Check sheet for the modelled part. Datum: model origin and axes. Units: mm. Face numbers are marked on the shaded views. A direction names the side the tool comes from. Coordinates: 2 decimals unless noted, no trailing zeros. Order: outer loops, then holes, each group sorted by start corner. A loop starts at its lowest first (then second) coordinate and runs counter-clockwise, first axis right, second up.
1. Thickness scan on line 1 (X direction, y = 1.75, z = 6.25); line 2 (X direction, y = -1.5, z = 2.75) (3 decimals); line 3 (Y direction, x = -7.25, z = 4). Record the ranges inside material, lowest first.
2. Cross-section at A-A (z = 7). Enter the section's corners in (x, y) (3 decimals).
3. Cross-section at B-B (x = 7.25). Enter the section's corners in (y, z).
4. Gauge pin test, flat ends, axial feed: pin 1 Ø2 at (y, z) = (2.5, 10) entering from +X; pin 2 Ø2 at (y, z) = (-4, 13) entering from -X; pin 3 Ø2 at (x, y) = (-6, 1) entering from +Z. Record the tip position at first contact, or that the pin passes through.
5. Draft check along Y on the marked faces 1, 2 and 3. Enter one of: released by +Y, released by -Y, zero draft, split by the parting line, or undercut.
6. Set-up check for the marked faces 4, 5 and 6: record each of +Z, -Z, +X, -X, +Y, -Y from which the full face is reachable in a straight line by a thin tool's end or side.
7. Cross-section at D-D (y = -3). Enter the section's corners in (x, z) (3 decimals).
8. Cross-section at C-C (z = 13.25). Enter the section's corners in (x, y).
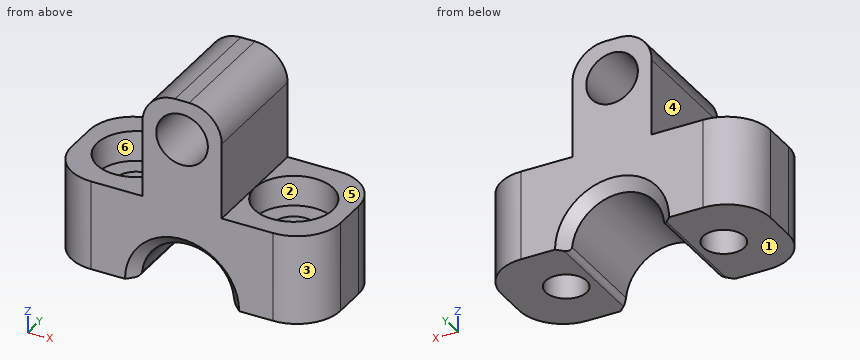
```python
from build123d import *

# Parameters (mm, degrees)
CROQUIS1_W                                           = 24.75
CROQUIS1_H                                           = 11
SALIENTE_EXTRUIR1_DEPTH                              = 8.25
REFRENTADO_PARA_TORNILLO_CON_CABEZA_HEXA_D           = 3.78
REFRENTADO_PARA_TORNILLO_CON_CABEZA_HEXA_DEPTH       = 8.25
REFRENTADO_PARA_TORNILLO_CON_CABEZA_HEXA_CBORE_D     = 7.2
REFRENTADO_PARA_TORNILLO_CON_CABEZA_HEXA_CBORE_DEPTH = 2.79
DI_METRO_DE_TALADRO_8_5_8_5_1_D                      = 8.5
DI_METRO_DE_TALADRO_8_5_8_5_1_DEPTH                  = 11
CHAFL_N1_SIZE                                        = 1
REDONDEO1_R                                          = 0.5
REDONDEO2_R                                          = 4
CROQUIS6_W                                           = 7.3
CROQUIS6_H                                           = 11
SALIENTE_EXTRUIR3_DEPTH                              = 10
CROQUIS7_R                                           = 2.375
CORTAR_EXTRUIR1_DEPTH                                = 6.5000001
CORTAR_EXTRUIR1_DEPTH_BACK                           = 6.5000001
REDONDEO3_R                                          = 3


with BuildPart() as part:
    # Croquis1 → Saliente-Extruir1 (new body)
    with BuildSketch(Plane(origin=(0, 0, 0), x_dir=(-1, 0, 0), z_dir=(0, 0, -1))):
        Rectangle(CROQUIS1_W, CROQUIS1_H)
    extrude(amount=-SALIENTE_EXTRUIR1_DEPTH)

    # Refrentado para tornillo con cabeza hexagonal de M3.51
    with Locations(Plane.XY.offset(8.25)):
        with Locations((-7.25, 0), (7.25, 0)):
            CounterBoreHole(REFRENTADO_PARA_TORNILLO_CON_CABEZA_HEXA_D / 2, REFRENTADO_PARA_TORNILLO_CON_CABEZA_HEXA_CBORE_D / 2, REFRENTADO_PARA_TORNILLO_CON_CABEZA_HEXA_CBORE_DEPTH, depth=REFRENTADO_PARA_TORNILLO_CON_CABEZA_HEXA_DEPTH)

    # Diámetro de taladro Ø8.5 (8.5)1
    with Locations(Plane(origin=(0, 5.5, 0), x_dir=(1, 0, 0), z_dir=(0, 1, 0))):
        with Locations((0, 0)):
            Hole(DI_METRO_DE_TALADRO_8_5_8_5_1_D / 2, depth=DI_METRO_DE_TALADRO_8_5_8_5_1_DEPTH)

    # Chaflán1
    chafl_n1_edges = [part.edges().sort_by_distance(p)[0] for p in [
        (0, 5.5, 4.25),
        (0, -5.5, 4.25),
    ]]
    chamfer(chafl_n1_edges, length=CHAFL_N1_SIZE)

    # Redondeo1
    redondeo1_edges = [part.edges().sort_by_distance(p)[0] for p in [
        (4.25, 0, 0),
        (-4.25, 0, 0),
    ]]
    fillet(redondeo1_edges, radius=REDONDEO1_R)

    # Redondeo2
    redondeo2_edges = [part.edges().sort_by_distance(p)[0] for p in [
        (-12.375, 5.5, 4.125),
        (-12.375, -5.5, 4.125),
        (12.375, -5.5, 4.125),
        (12.375, 5.5, 4.125),
    ]]
    fillet(redondeo2_edges, radius=REDONDEO2_R)

    # Croquis6 → Saliente-Extruir3 (add)
    with BuildSketch(Plane.XY.offset(8.25)):
        Rectangle(CROQUIS6_W, CROQUIS6_H)
    extrude(amount=SALIENTE_EXTRUIR3_DEPTH)

    # Croquis7 → Cortar-Extruir1 (cut, two sides)
    with BuildSketch(Plane(origin=(0, 0, 0), x_dir=(1, 0, 0), z_dir=(0, 1, 0))) as cortar_extruir1_sk:
        with Locations((0, -14.6)):
            Circle(CROQUIS7_R)
    extrude(amount=CORTAR_EXTRUIR1_DEPTH, mode=Mode.SUBTRACT)
    extrude(cortar_extruir1_sk.sketch, amount=-CORTAR_EXTRUIR1_DEPTH_BACK, mode=Mode.SUBTRACT)

    # Redondeo3
    redondeo3_edges = [part.edges().sort_by_distance(p)[0] for p in [
        (3.65, 0, 18.25),
        (-3.65, 0, 18.25),
    ]]
    fillet(redondeo3_edges, radius=REDONDEO3_R)


solid = part.part
```
Data:
1. line 1: x = -12.37 to -10.4, -4.1 to 4.1, 10.4 to 12.37
1. line 2: x = -12.375 to -8.4, -6.1 to -3.24, 3.24 to 6.1, 8.4 to 12.375
1. line 3: y = -5.5 to -1.89, 1.89 to 5.5
2. outline: (-12.375, -1.5) arc R4 ccw to (-8.375, -5.5) - (8.375, -5.5) arc R4 ccw to (12.375, -1.5) - (12.375, 1.5) arc R4 ccw to (8.375, 5.5) - (-8.375, 5.5) arc R4 ccw to (-12.375, 1.5) - close; hole circle Ø7.2 at (-7.25, 0); hole circle Ø7.2 at (7.25, 0)
3. outline: (-5.5, 0) - (-1.89, 0) - (-1.89, 5.46) - (-3.6, 5.46) - (-3.6, 8.25) - (-5.5, 8.25) - close; (1.89, 0) - (5.5, 0) - (5.5, 8.25) - (3.6, 8.25) - (3.6, 5.46) - (1.89, 5.46) - close
4. pin 1: stops at x = 3.65
4. pin 2: stops at x = -3.65
4. pin 3: stops at z = 5.46
5. face 1: zero draft
5. face 2: undercut
5. face 3: released by -Y
6. face 4: +Z, -X, +Y, -Y
6. face 5: +Z, +X, +Y, -Y
6. face 6: +Z
7. outline: (-12.083, 0) - (-4.724, 0) arc R0.5 ccw to (-4.226, 0.447) arc R4.25 cw to (4.226, 0.447) arc R0.5 ccw to (4.724, 0) - (12.083, 0) - (12.083, 8.25) - (9.24, 8.25) - (9.24, 5.46) - (5.26, 5.46) - (5.26, 8.25) - (3.65, 8.25) - (3.65, 15.25) arc R3 ccw to (0.65, 18.25) - (-0.65, 18.25) arc R3 ccw to (-3.65, 15.25) - (-3.65, 8.25) - (-5.26, 8.25) - (-5.26, 5.46) - (-9.24, 5.46) - (-9.24, 8.25) - (-12.083, 8.25) - close; hole circle Ø4.75 at (0, 14.6)
8. outline: (-3.65, -5.5) - (-1.95, -5.5) - (-1.95, 5.5) - (-3.65, 5.5) - close; (1.95, -5.5) - (3.65, -5.5) - (3.65, 5.5) - (1.95, 5.5) - close
